Read the model definition and answer for the solid it produces. Units are mm, in the model's axes. Face numbers are marked on the shaded views. A direction names the side the tool comes from. Coordinates: 2 decimals unless noted, no trailing zeros. Order: outer loops, then holes, each group sorted by start corner. A loop starts at its lowest first (then second) coordinate and runs counter-clockwise, first axis right, second up. Notation, with made-up numbers: M 12.5,68 L 47.5,68 A27 ccw 47.5,90 Z; hole C 14.5,2.5 d9. An arc over 180 degrees is marked long. One line per question, with ' | ' between items. Start each with the question number.
1) Consider probe 1 along Z at (x, y) = (31, -14); probe 2 along Y at (x, z) = (23, -44.3); probe 3 along Z at (x, y) = (-10, -18). Determine where each line is inside the solid, lowest interval first.
2) The mould has two halves that part along Z. Classify the marked faces 1, 2, 3 and 4: +Z half, -Z half, draft (parallel to the pull), parting line (faces both ways), or undercut.
3) Find section C-C, the plane x = 20.5. Write down the section's boundary in (y, z).
4) Find section B-B, the plane y = 0. Count the separate pieces of the cut face and the enclosed holes in it, plus the area to 4 significant figures.
5) Find section A-A, the plane z = -26.5. Write down the section's boundary in (x, y), plus the area to 3 significant figures.
6) A tool of negligible diameter and unlimited length cuts with its end or side. For the marked faces 5, 6, 7 and 8, from which of +Z, -Z, +X, -X, +Y, -Y can it reach the whole face along a straight path? Write none if from no direction.
7) Find section D-D, the plane y = 10.5. Write down the section's boundary in (x, z), plus the area to 3 significant figures.
8) Given P1, Ø2, axis at x = -31, y = -0.5, coming from the -Z side; P2, Ø6, axis at y = 17.5, z = -20, coming from the +X side; P3, Ø8, axis at y = 16.5, z = -19.5, coming from the -X side, each flat-ended and moving along its own axis, determine where each tip first touches the part or whether it passes through.
from build123d import *

# Parameters (mm, degrees)
BOSS_EXTRUDE1_DEPTH = 8.5
SKETCH2_R           = 20.5
CUT_EXTRUDE1_DEPTH  = 4.25
SKETCH3_R           = 20.5
CUT_EXTRUDE2_DEPTH  = 4.25
SKETCH4_R           = 6.25
CUT_EXTRUDE3_DEPTH  = 5.25
SKETCH5_R           = 6.25
BOSS_EXTRUDE2_DEPTH = 4.25
SKETCH6_W           = 13.503846382
SKETCH6_H           = 7.5
BOSS_EXTRUDE3_DEPTH = 38


with BuildPart() as part:
    # Sketch1 → Boss-Extrude1 (new body)
    with BuildSketch(Plane.XY):
        with BuildLine():
            Line((-23, 20), (23, 20))
            ThreePointArc((23, 20), (43, 0), (23, -20))
            Line((23, -20), (-23, -20))
            ThreePointArc((-23, -20), (-43, 0), (-23, 20))
        make_face()
    extrude(amount=BOSS_EXTRUDE1_DEPTH)

    # Sketch2 → Cut-Extrude1 (cut)
    with BuildSketch(Plane(origin=(0, 0, 0), x_dir=(-1, 0, 0), z_dir=(0, 0, -1))):
        with Locations((-23, 0)):
            Circle(SKETCH2_R)
    extrude(amount=-CUT_EXTRUDE1_DEPTH, mode=Mode.SUBTRACT)

    # Sketch3 → Cut-Extrude2 (cut)
    with BuildSketch(Plane.XY.offset(8.5)):
        with Locations((-23, 0)):
            Circle(SKETCH3_R)
    extrude(amount=-CUT_EXTRUDE2_DEPTH, mode=Mode.SUBTRACT)

    # Sketch4 → Cut-Extrude3 (cut, through all)
    with BuildSketch(Plane(origin=(0, 0, 4.25), x_dir=(-1, 0, 0), z_dir=(0, 0, -1))):
        with Locations((-23, 0)):
            Circle(SKETCH4_R)
    extrude(amount=-CUT_EXTRUDE3_DEPTH, mode=Mode.SUBTRACT)

    # Sketch5 → Boss-Extrude2 (add)
    with BuildSketch(Plane.XY.offset(4.25)):
        with Locations((-23, 0)):
            Circle(SKETCH5_R)
    extrude(amount=BOSS_EXTRUDE2_DEPTH)

    # Sketch6 → Boss-Extrude3 (add)
    with BuildSketch(Plane(origin=(0, 0, 0), x_dir=(-1, 0, 0), z_dir=(0, 0, -1))):
        with Locations((0, 16.25)):
            Rectangle(SKETCH6_W, SKETCH6_H)
    boss_extrude3 = extrude(amount=BOSS_EXTRUDE3_DEPTH)

    # Mirror1: Boss-Extrude3 across plane
    add(boss_extrude3.mirror(Plane.ZX))

    # Зеркальное отражение1: part across plane


with BuildPart() as part_1:
    add(part.part)
    add(part.part.mirror(Plane.XY.offset(-19)))


solid = part_1.part
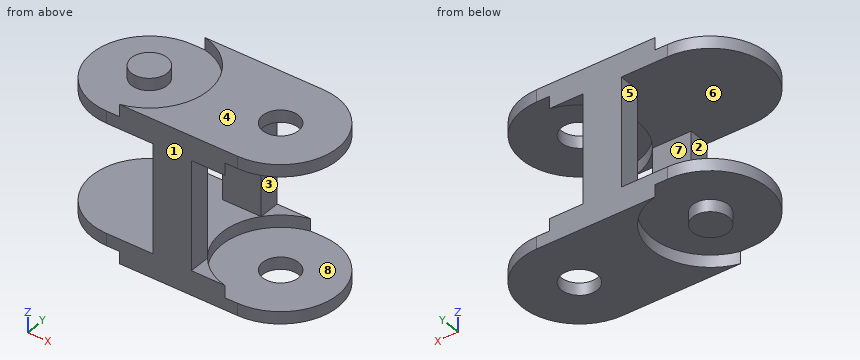
Report:
1) probe 1: z = -46.5 to -42.25, 4.25 to 8.5 | probe 2: y = -20 to -6.25, 6.25 to 20 | probe 3: z = -46.5 to -38, 0 to 8.5
2) face 1: draft | face 2: undercut | face 3: undercut | face 4: +Z half
3) outline: M -20,-46.5 L -5.73,-46.5 L -5.73,-42.25 L -20,-42.25 Z; M -20,4.25 L -5.73,4.25 L -5.73,8.5 L -20,8.5 Z; M 5.73,-46.5 L 20,-46.5 L 20,-42.25 L 5.73,-42.25 Z; M 5.73,4.25 L 20,4.25 L 20,8.5 L 5.73,8.5 Z
4) separate pieces: 4 | enclosed holes: 0 | area: 773.5 mm^2
5) outline: M -6.75,-20 L 6.75,-20 L 6.75,-12.5 L -6.75,-12.5 Z; M -6.75,12.5 L 6.75,12.5 L 6.75,20 L -6.75,20 Z | area: 203 mm^2
6) face 5: -X, +Y, -Y | face 6: -X | face 7: +X, -X | face 8: +X
7) outline: M -40.02,-42.25 L -5.39,-42.25 L -5.39,-46.5 L 40.02,-46.5 L 40.02,-42.25 L 5.39,-42.25 L 5.39,-38 L -40.02,-38 Z; M -40.02,0 L 5.39,0 L 5.39,4.25 L 40.02,4.25 L 40.02,8.5 L -5.39,8.5 L -5.39,4.25 L -40.02,4.25 Z | area: 772 mm^2
8) P1: stops at z = -42.25 | P2: stops at x = 6.75 | P3: stops at x = -6.75
